Model file for the job. Use its own axes, mm. Round coordinates to 2 decimals unless told otherwise and drop trailing zeros. Order: outer loops, then holes, each group sorted by start corner. A loop starts at its lowest first (then second) coordinate and runs counter-clockwise, first axis right, second up. Notation, with made-up numbers: (-27, 9.5) -> (21, 9.5) arc R23 cw to (21, 36.5) -> close; hole circle Ø8 at (-18.5, 15). An arc over 180 degrees is marked (long way). Put each result on its own line as item: value. Start each with the question number.
Q1. Pull direction Y, two halves, no side cores. Call faces 1 (the face through (-10.316, -7.91, 3.951)), 2 (the face through (3, -5, 8)), 3 (the face through (-1.08, -4.88, 4.05)): released by +Y, released by -Y, zero draft, split by the parting line, or undercut.
Q2. Cut at C-C, the plane z = 2.25. List the corners of the cut face in (x, y), and give its area (3 significant figures).
Q3. Flat gauge pins, fed straight in: P1, Ø2, axis at y = 5, z = 3.5, coming from the +X side; P2, Ø5, axis at x = -1.5, y = 0.5, coming from the +Z side. Where does each tip first touch, or does it go through?
Q4. Cut at A-A, the plane x = 0. List the corners of the cut face in (y, z).
Q5. Probe L1, parallel to Y at x = 0, z = 2.5; L2, parallel to Y at x = 4.5, z = 4.75; L3, parallel to X at y = 3.5, z = 4.75. List the from-to ranges inside material, lowest first.
from build123d import *

# Parameters (mm, degrees)
SKETCH1_R           = 13
BOSS_EXTRUDE1_DEPTH = 8
SKETCH2_R           = 5
CUT_EXTRUDE1_DEPTH  = 8
CHAMFER1_SIZE       = 0.5


with BuildPart() as part:
    # Sketch1 → Boss-Extrude1 (new body)
    with BuildSketch(Plane.XY):
        Circle(SKETCH1_R)
    extrude(amount=BOSS_EXTRUDE1_DEPTH)

    # Sketch2 → Cut-Extrude1 (cut)
    with BuildSketch(Plane.XY.offset(8)):
        Circle(SKETCH2_R)
    extrude(amount=-CUT_EXTRUDE1_DEPTH, mode=Mode.SUBTRACT)

    # Chamfer1
    chamfer1_edges = [part.edges().sort_by_distance(p)[0] for p in [
        (-13, 0, 0),
        (-13, 0, 8),
        (-5, 0, 0),
        (-5, 0, 8),
    ]]
    chamfer(chamfer1_edges, length=CHAMFER1_SIZE)


solid = part.part
Ans:
1. face 1: split by the parting line
1. face 2: zero draft
1. face 3: undercut
2. outline: circle Ø26 at (0, 0); hole circle Ø10 at (0, 0)
2. area: 452 mm^2
3. P1: stops at x = 12.37
3. P2: passes through
4. outline: (-13, 0.5) -> (-12.5, 0) -> (-5.5, 0) -> (-5, 0.5) -> (-5, 7.5) -> (-5.5, 8) -> (-12.5, 8) -> (-13, 7.5) -> close; (5, 0.5) -> (5.5, 0) -> (12.5, 0) -> (13, 0.5) -> (13, 7.5) -> (12.5, 8) -> (5.5, 8) -> (5, 7.5) -> close
5. L1: y = -13 to -5, 5 to 13
5. L2: y = -12.2 to -2.18, 2.18 to 12.2
5. L3: x = -12.52 to -3.57, 3.57 to 12.52
